Could you check a few things on this model? Use its own coordinates, in mm. Face numbers are marked on the shaded views. Coordinates: 2 decimals unless noted, no trailing zeros. Write each loop counter-clockwise with the first axis right and the second up, starting at its lowest first coordinate (ties: lowest second). Pieces come first, ordered by that corner, then holes.
Item 1: I want a section at D-D on y = -20. Please give me the cut outline in (x, z), then the cut area to 3 significant figures.
Item 2: I want a section at A-A on z = -2. Please give me the cut outline in (x, y) (3 decimals), then the cut area to 3 significant figures.
Item 3: I want a section at B-B on y = 4. Please give me the cut outline in (x, z).
Item 4: If I drill on probe 1 along X at (y, z) = (5, -2.75); probe 2 along Z at (x, y) = (-2.5, -25.5); probe 3 along X at (y, z) = (1, -0.5), over which ranges is the centre line in solid material (lowest first)?
Item 5: For P1, Ø1.5, axis at x = -26.5, z = -5.5, coming from the +Y side; P2, Ø2.5, axis at y = 4, z = -4, coming from the +X side; P3, Ø1, axis at y = 13, z = -1, coming from the -X side; P4, Ø2, axis at x = -7, y = -12, coming from the -Z side, each with a flat end and sliding along its axis, tell me the tip position at first contact or that it passes through.
Item 6: I want a section at C-C on x = -2. Please give me the cut outline in (y, z).
Item 7: Thinking about a two-plate mould opening in X: for the marked faces 1 and 2, which applies, +X half, -X half, draft (parallel to the pull), parting line (faces both ways), or undercut?
Autodesk Inventor part; units mm, degrees
ref_plane "YZ Plane" through (0, 0, 0) normal (1, 0, 0) x (0, 1, 0)
ref_plane "XZ Plane" through (0, 0, 0) normal (0, 1, 0) x (-1, 0, 0)
ref_plane "XY Plane" through (0, 0, 0) normal (0, 0, 1) x (1, 0, 0)
ref_plane "Work Plane1" through (0, 0, 0) normal (0, 0, 1) x (1, 0, 0)
sketch "Sketch1" plane through (0, 0, 0) normal (0, 0, 1) x (1, 0, 0)
  arc A0 (14.605, -35.56) -> (17.78, -32.385) centre (14.605, -32.385) ccw
  line L0 (17.78, -32.385) -> (17.78, 33.985)
  arc A1 (17.78, 33.985) -> (14.605, 37.16) centre (14.605, 33.985) ccw
  line L1 (14.605, 37.16) -> (-29.845, 37.16)
  arc A2 (-29.845, 37.16) -> (-33.02, 33.985) centre (-29.845, 33.985) ccw
  line L2 (-33.02, 33.985) -> (-33.02, -32.385)
  arc A3 (-33.02, -32.385) -> (-29.845, -35.56) centre (-29.845, -32.385) ccw
  line L3 (-29.845, -35.56) -> (14.605, -35.56)
  line L4 (13.105, -34.06) -> (-28.345, -34.06)
  arc A4 (-31.52, -30.885) -> (-28.345, -34.06) centre (-28.345, -30.885) ccw
  line L5 (-31.52, -30.885) -> (-31.52, 30.885)
  arc A5 (-28.345, 34.06) -> (-31.52, 30.885) centre (-28.345, 30.885) ccw
  line L6 (-28.345, 34.06) -> (13.105, 34.06)
  arc A6 (16.28, 30.885) -> (13.105, 34.06) centre (13.105, 30.885) ccw
  line L7 (16.28, 30.885) -> (16.28, -30.885)
  arc A7 (13.105, -34.06) -> (16.28, -30.885) centre (13.105, -30.885) ccw
  point P0 (0, 0)
extrude "Extrusion1" add sketch "Sketch1" along normal blind 1 contours L3 A3 L2 A2 L1 A1 L0 A0 | L4 A4 L5 A5 L6 A6 L7 A7
ref_plane "Work Plane2" through (-29.845, 0.8, 0) normal (0, 1, 0) x (1, 0, 0)
sketch "Sketch3" plane through (-29.845, 0.8, 0) normal (0, 1, 0) x (1, 0, 0)
  line L0 (46.125, 31.5) -> (46.125, 0)
  line L1 (47.625, 5) -> (47.625, 7)
  line L2 (46.125, 5) -> (47.625, 5)
  line L3 (46.125, 7) -> (46.125, 5)
  line L4 (46.125, 7) -> (47.625, 7)
  line L5 (43.375, 0) -> (43.375, 6.8424)
  line L6 (43.375, 6.8424) -> (45.775, 6.8424)
  line L7 (45.775, 6.8424) -> (47.371, 6.0831)
  line L8 (47.371, 6.0831) -> (47.371, 5.3048)
  line L9 (47.371, 5.3048) -> (45.875, 5.3048)
  line L10 (45.875, 5.3048) -> (45.875, 0)
  line L11 (44.45, 0) -> (0, 0)
  line L12 (43.375, 0) -> (45.875, 0)
  point P0 (29.845, 0)
  dimension "d17" = 2.5
  dimension "d18" = 0.25
  dimension "d19" = 0.254
  dimension "d20" = 0.3048
  dimension "d21" = 0.1576
  dimension "d23" = 1.496
  dimension "d25" = 115.445
  dimension "d26" = 0.7783
extrude "Extrusion3" add sketch "Sketch3" along normal mid plane 24.13 contours L7 L8 L9 L0 | L0 L9 L10 L12 L11 L5 L6 L7
ref_plane "Work Plane3" through (-7.62, -32.385, 0) normal (-1, 0, 0) x (0, 0, 1)
mirror "Mirror1" about plane through (-7.62, -32.385, 0) normal (-1, 0, 0) of "Extrusion3"
fillet "Fillet1" radius 1.27 1 edges at (13.53, 0.8, 0)
fillet "Fillet2" radius 1.27 1 edges at (-28.77, 0.8, 0)
properties part number "lidV2"
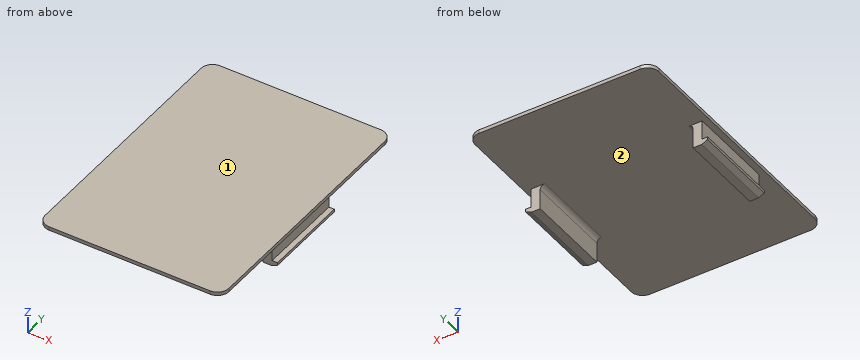
Response values:
1. outline: (-33.02, 0) - (17.78, 0) - (17.78, 1) - (-33.02, 1) - close
1. area: 50.8 mm2
2. outline: (-31.27, -11.265) - (-28.77, -11.265) - (-28.77, 12.865) - (-31.27, 12.865) - close; (13.53, -11.265) - (16.03, -11.265) - (16.03, 12.865) - (13.53, 12.865) - close
2. area: 121 mm2
3. outline: (-33.02, 0) - (-31.27, 0) - (-31.27, -5.3) - (-32.77, -5.3) - (-32.77, -6.08) - (-31.17, -6.84) - (-28.77, -6.84) - (-28.77, -1.27) arc R1.27 cw to (-27.5, 0) - (12.26, 0) arc R1.27 cw to (13.53, -1.27) - (13.53, -6.84) - (15.93, -6.84) - (17.53, -6.08) - (17.53, -5.3) - (16.03, -5.3) - (16.03, 0) - (17.78, 0) - (17.78, 1) - (-33.02, 1) - close
4. probe 1: x = -31.27 to -28.77, 13.53 to 16.03
4. probe 2: z = 0 to 1
4. probe 3: x = -31.27 to -28.51, 13.27 to 16.03
5. P1: passes through
5. P2: stops at x = 16.03
5. P3: stops at x = -31.27
5. P4: stops at z = 0
6. outline: (-35.56, 0) - (37.16, 0) - (37.16, 1) - (-35.56, 1) - close
7. face 1: draft
7. face 2: undercut
